from build123d import *

# Parameters (mm, degrees)
F0_W     = 88.9
F0_H     = 17.78
F0_R     = 1.5875
F0_R_2   = 3.175
F1_DEPTH = 3.175
F2_R     = 3.175
F3_DEPTH = 20.32


with BuildPart() as f1:
    # F0 (on Front) → F1 (new body)
    with BuildSketch(Plane.XZ):
        with Locations((-0.217237, -27.299299)):
            Rectangle(F0_W, F0_H)
        with Locations((-18.632237, -29.130639)):
            Circle(F0_R, mode=Mode.SUBTRACT)
        with Locations((-37.682237, -26.664299)):
            Circle(F0_R_2, mode=Mode.SUBTRACT)
        with Locations((-2.249237, -25.394299)):
            Circle(F0_R, mode=Mode.SUBTRACT)
        with Locations((34.707763, -26.664299)):
            Circle(F0_R_2, mode=Mode.SUBTRACT)
    extrude(amount=F1_DEPTH)

    # F2 (on face) → F3 (join)
    with BuildSketch(Plane(origin=(0, 0, 0), x_dir=(-1, 0, 0), z_dir=(0, 1, 0))):
        with Locations((-34.707763, -26.664299)):
            Circle(F2_R)
        with Locations((37.682237, -26.664299)):
            Circle(F2_R)
    extrude(amount=-F3_DEPTH)


solid = f1.part
The model under review builds one solid part; all positions refer to its coordinate system, in mm. A direction names the side the tool comes from. Coordinates: 2 decimals unless noted, no trailing zeros. Write each loop counter-clockwise with the first axis right and the second up, starting at its lowest first coordinate (ties: lowest second). Pieces come first, ordered by that corner, then holes. Notation, with made-up numbers: (87.25, 48.25) -> (117.25, 48.25) arc R20 cw to (117.25, 87.25) -> close; hole circle Ø10 at (-16, -6.75). An arc over 180 degrees is marked (long way). Answer in a Markdown table with one row per item.
1. Clearance check with flat-ended pins moving along their axes: pin 1 Ø9 at (x, z) = (-15, -27) entering from -Y (3 decimals); pin 2 Ø5 at (y, z) = (-10, -22) entering from -X; pin 3 Ø5 at (y, z) = (-9, -27) entering from -X. State where each tip first meets the part, or that it passes through.
Answers below:
| item | result |
|---|---|
| pin 1 | stops at y = -3.175 |
| pin 2 | stops at x = -40.01 |
| pin 3 | stops at x = -40.86 |
2. We need section C-C, the plane x = 5.5. State the section outline as (y, z) points (3 decimals), and give its area (3 significant figures).
Answers below:
| item | result |
|---|---|
| outline | (-3.175, -36.189) -> (0, -36.189) -> (0, -18.409) -> (-3.175, -18.409) -> close |
| area | 56.5 mm^2 |
3. We need section B-B, the plane y = -11.5. State the section outline as (x, z) points (3 decimals).
Answers below:
| item | result |
|---|---|
| outline | circle Ø6.35 at (-37.682, -26.664); circle Ø6.35 at (34.708, -26.664) |
4. For faces 1 (the cylindrical face through (-2.593, -1.565, -26.944)), 2 (the cylindrical face through (-39.15, -11.63, -29.48)), list the 3-axis set-ups (+Z, -Z, +X, -X, +Y, -Y) from which the entire face can be reached by the end or side of a thin tool; tool diameter is ignored.
Answers below:
| item | result |
|---|---|
| face 1 | +Y, -Y |
| face 2 | -Y |
5. Draft analysis for pull direction Z (two halves, no side actions). For faces 3 (the flat face through (44.233, -2, -27)), 4 (the cylindrical face through (31.775, -11.627, -27.88)), 5 (the flat face through (-1, -2, -18.409)), 6 (the cylindrical face through (-18.98, -1.57, -30.68)), state which applies: +Z half, -Z half, draft (parallel to the pull), parting line (faces both ways), or undercut.
Answers below:
| item | result |
|---|---|
| face 3 | draft |
| face 4 | parting line |
| face 5 | +Z half |
| face 6 | undercut |
6. We need section A-A, the plane z = -20.5. State the section outline as (x, y) points (3 decimals).
Answers below:
| item | result |
|---|---|
| outline | (-44.667, -3.175) -> (44.233, -3.175) -> (44.233, 0) -> (-44.667, 0) -> close |
7. Wall thickness on probe 1 along X at (y, z) = (-11.75, -27); probe 2 along Y at (x, z) = (2, -34) (3 decimals); probe 3 along X at (y, z) = (-17, -27.75): over which ranges is each line inside the solid? List them lowest first. Write a range as [from, to].
Answers below:
| item | result |
|---|---|
| probe 1 | x = [-40.84, -34.53], [31.55, 37.86] |
| probe 2 | y = [-3.175, 0] |
| probe 3 | x = [-40.67, -34.7], [31.72, 37.69] |
